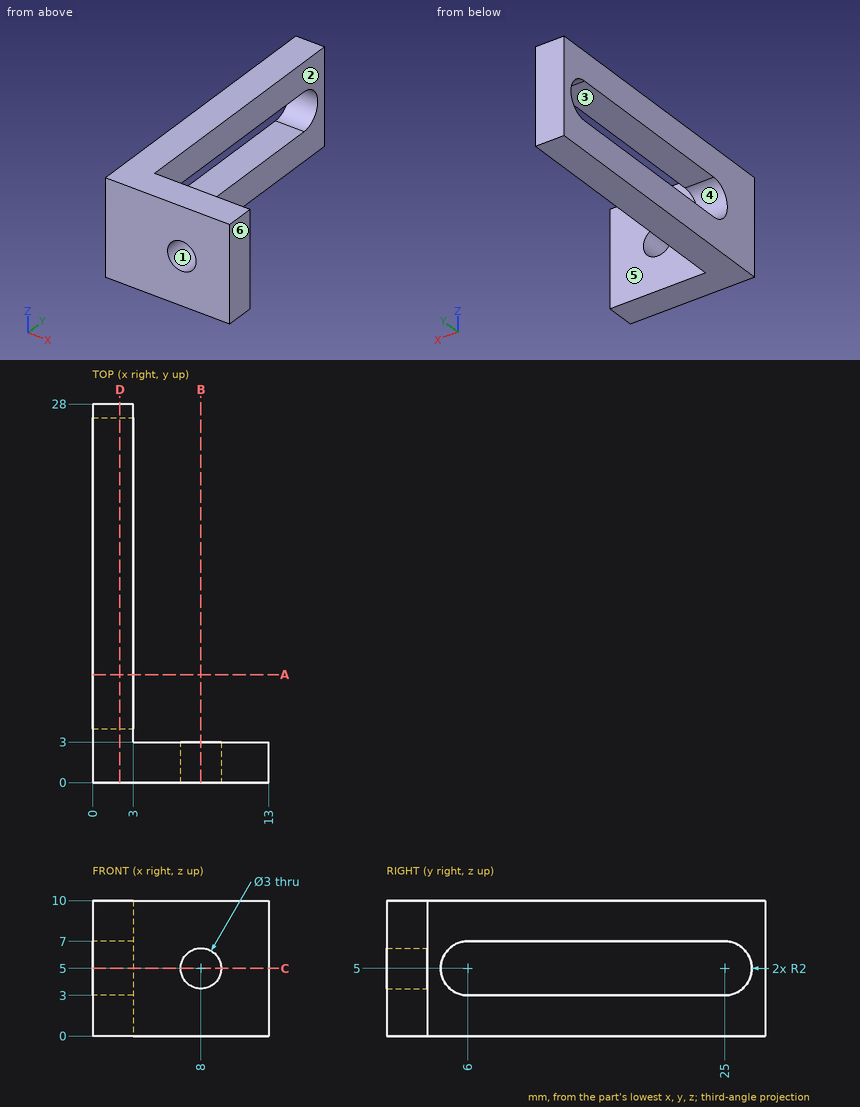
For this review, use the dimensioned drawing (mm, ordinates from the lowest corner) and the shaded views. A direction names the side the tool comes from. Round coordinates to 2 decimals unless told otherwise and drop trailing zeros. Loops run counter-clockwise (first coordinate to the right, second up) from the corner with the lowest first, then second, coordinate; pieces in that order, holes last. Notation, with made-up numbers: (6.5, 75.25) -> (11.5, 75.25) arc R19 cw to (11.5, 104.25) -> close; hole circle Ø10 at (0.5, 78.25). An arc over 180 degrees is marked (long way). Write item = value, one per line. Start each with the question number.
Item 1: To check wall thickness, follow L1, parallel to Z at x = 8, y = 1; L2, parallel to X at y = 0.9, z = 5; L3, parallel to X at y = 8, z = 9. State the ranges of each line that lie inside material, in increasing order.
Item 2: Take a section at C-C on z = 5. Give the boundary of the cut face in (x, y), plus the area to 3 significant figures.
Item 3: Insertion check: pin 1 (4 mm diameter, centred on y = 13.5, z = 3, fed in from +X); pin 2 (5 mm diameter, centred on x = 8, z = 5, fed in from -Y); pin 3 (2 mm diameter, centred on x = 10, z = 3, fed in from +Y); pin 4 (3 mm diameter, centred on x = 6, y = 7.5, fed in from +Z). Each pin has a flat end and moves straight along its axis. Give the tip position at first contact, or say it passes through.
Item 4: Take a section at A-A on y = 8. Give the boundary of the cut face in (x, z), plus the area to 3 significant figures.
Item 5: Mouldability with a two-part tool opening along X and no side actions: class the marked faces 1, 2 and 3 as released by +X, released by -X, zero draft, split by the parting line, or undercut.
Item 6: Take a section at D-D on x = 2. Give the boundary of the cut face in (y, z).
Item 7: Take a section at B-B on x = 8. Give the boundary of the cut face in (y, z).
Item 8: For the marked faces 4, 5 and 6, list the 3-axis set-ups (+Z, -Z, +X, -X, +Y, -Y) from which the entire face can be reached by the end or side of a thin tool; tool diameter is ignored.
Result:
q1.L1 = 0 to 3.5, 6.5 to 10
q1.L2 = 0 to 6.5, 9.5 to 13
q1.L3 = 0 to 3
q2.outline = (0, 0) -> (6.5, 0) -> (6.5, 3) -> (3, 3) -> (3, 4) -> (0, 4) -> close; (0, 27) -> (3, 27) -> (3, 28) -> (0, 28) -> close; (9.5, 0) -> (13, 0) -> (13, 3) -> (9.5, 3) -> close
q2.area = 36.0 mm²
q3.pin_1 = 3
q3.pin_2 = 0
q3.pin_3 = 3
q3.pin_4 = through
q4.outline = (0, 0) -> (3, 0) -> (3, 3) -> (0, 3) -> close; (0, 7) -> (3, 7) -> (3, 10) -> (0, 10) -> close
q4.area = 18.0 mm²
q5.face_1 = undercut
q5.face_2 = released by +X
q5.face_3 = zero draft
q6.outline = (0, 0) -> (28, 0) -> (28, 10) -> (0, 10) -> close; hole (6, 3) -> (25, 3) arc R2 ccw to (25, 7) -> (6, 7) arc R2 ccw to start
q7.outline = (0, 0) -> (3, 0) -> (3, 3.5) -> (0, 3.5) -> close; (0, 6.5) -> (3, 6.5) -> (3, 10) -> (0, 10) -> close
q8.face_4 = +X, -X
q8.face_5 = +Z, -Z, +X, +Y
q8.face_6 = +Z, -Z, +X, +Y, -Y
